The listing builds one solid part. Answer for the finished solid, in the listing's coordinates (mm). A direction names the side the tool comes from. Round coordinates to 2 decimals unless told otherwise and drop trailing zeros. Write each loop counter-clockwise with the first axis right and the second up, starting at its lowest first coordinate (ties: lowest second). Pieces come first, ordered by that corner, then holes. Notation, with made-up numbers: (45, 41) - (72, 41) arc R11 cw to (72, 50) - close; hole circle Ø11 at (-17.75, 24.5). An arc over 180 degrees is marked (long way). Return JSON: item names as keys, results as strings. Group by question number.
(1) Section B-B, the plane z = -3.25 is taken. Write down the section's boundary in (x, y), then the cut area to 3 significant figures.
(2) Determine the mould class of faces 3 (the flat face through (-12.45, -12.3, -0.14)), 4 (the flat face through (1, -54.428, -2)), 5 (the flat face through (41.704, 31, 0)), 6 (the cylindrical face through (-46.7, -3.73, 2.84)) for opening direction Y: +Y half, -Y half, draft (parallel to the pull), parting line (faces both ways), or undercut.
(3) Each of these flat-tipped pins is pushed along its axis until it touches: pin 1 (4 mm diameter, centred on x = 34.5, z = 0.5, fed in from -Y); pin 2 (1 mm diameter, centred on y = -4, z = 1.5, fed in from -X). Where does it stop, or does it pass through?
(4) Which of the six approach directions +Z, -Z, +X, -X, +Y, -Y give full straight-line access (tool end or side, diameter ignored) to faces 1 (the flat face through (-12.3, 12.45, -0.14)), 2 (the cylindrical face through (0.9, -52.73, 2.84))?
(5) Find the intervals of material crossed by line 1 along X through (y, z) = (32.5, -0.25); line 2 along Y through (x, z) = (3, 0); line 3 along Y through (x, z) = (34, 2.5), in increasing order. Write a range as [from, to].
(6) Section C-C, the plane x = 14 is taken. Write down the section's boundary in (y, z), then the cut area to 3 significant figures.
(7) Section A-A, the plane y = 0.5 is taken. Write down the section's boundary in (x, z).
```python
from build123d import *

# Parameters (mm, degrees)
F0_W        = 100
F0_H        = 100
F1_DEPTH    = 4
F3_T1_DEPTH = 124.4948974279
F3_T3_DEPTH = 124.4948974279
F5_DEPTH    = 25
F4_W        = 10
F4_H        = 10
F6_DEPTH    = 25
F7_DEPTH    = 4.4


# Not quite as in the source:
# - a fillet or chamfer that OpenCascade refuses, or shapes differently, is made with other operations: its cross-section is extruded or revolved along the edge and cut away or added


with BuildPart() as f1:
    # F0 (on Top) → F1 (new body)
    with BuildSketch(Plane.XY):
        with Locations((1.60311535, -4.4280775759)):
            Rectangle(F0_W, F0_H)
    extrude(amount=F1_DEPTH)

    # F3: fillet of radius 5 on 4 edges, made by hand

    # F3_s2 → F3_t1 (cut)
    with BuildSketch(Plane.YZ.offset(-60.6443333639)):
        with BuildLine():
            ThreePointArc((-54.4280775759, 0), (-52.6913757505, 2.8729833462), (-49.5290980903, 4))
            Line((-49.5290980903, 4), (-54.4280775759, 4))
            Line((-54.4280775759, 4), (-54.4280775759, 0))
        make_face()
        with BuildLine():
            ThreePointArc((45.5719224241, 0), (43.8352205987, 2.8729833462), (40.6729429385, 4))
            Line((40.6729429385, 4), (45.5719224241, 4))
            Line((45.5719224241, 4), (45.5719224241, 0))
        make_face()
    extrude(amount=F3_T1_DEPTH, mode=Mode.SUBTRACT)

    # F3_s4 → F3_t3 (cut)
    with BuildSketch(Plane.XZ.offset(-57.819371138)):
        with BuildLine():
            ThreePointArc((51.60311535, 0), (49.8664135246, 2.8729833462), (46.7041358644, 4))
            Line((46.7041358644, 4), (51.60311535, 4))
            Line((51.60311535, 4), (51.60311535, 0))
        make_face()
        with BuildLine():
            ThreePointArc((-48.39688465, 0), (-46.6601828246, 2.8729833462), (-43.4979051644, 4))
            Line((-43.4979051644, 4), (-48.39688465, 4))
            Line((-48.39688465, 4), (-48.39688465, 0))
        make_face()
    extrude(amount=F3_T3_DEPTH, mode=Mode.SUBTRACT)

    # F2 (on face) → F5 (cut)
    with BuildSketch(Plane.XY.offset(4)):
        Polygon((-7.2487373415, -17.5), (7.2487373415, -17.5), (17.5, -7.2487373415), (17.5, 7.2487373415), (7.2487373415, 17.5), (-7.2487373415, 17.5), (-17.5, 7.2487373415), (-17.5, -7.2487373415), align=None)
    extrude(amount=-F5_DEPTH, mode=Mode.SUBTRACT)

    # F4 (on face) → F6 (cut)
    with BuildSketch(Plane.XY.offset(4)):
        with Locations((36.7041358644, 30.6729429385)):
            Rectangle(F4_W, F4_H)
    extrude(amount=-F6_DEPTH, mode=Mode.SUBTRACT)

    # F7 (add): a face of the model
    f7_faces = [f1.faces().sort_by_distance(p)[0] for p in [
        (1.60311535, -53.0138640135, 0),
    ]]
    extrude(f7_faces, amount=F7_DEPTH)


solid = f1.part
```
Working result:
{
 "1": {"outline": "(-48.4, -54.43) - (51.6, -54.43) - (51.6, 45.57) - (-48.4, 45.57) - close; hole (-17.5, -7.25) - (-7.25, -17.5) - (7.25, -17.5) - (17.5, -7.25) - (17.5, 7.25) - (7.25, 17.5) - (-7.25, 17.5) - (-17.5, 7.25) - close; hole (31.7, 25.67) - (41.7, 25.67) - (41.7, 35.67) - (31.7, 35.67) - close", "area": "8,890 mm^2"},
 "2": {"face 3": "undercut", "face 4": "-Y half", "face 5": "undercut", "face 6": "draft"},
 "3": {"pin 1": "stops at y = -54.43", "pin 2": "stops at x = -48.08"},
 "4": {"face 1": "+Z, -Z", "face 2": "+Z, +X, -X, -Y"},
 "5": {"line 1": "x = [-48.4, 31.7], [41.7, 51.6]", "line 2": "y = [-54.43, -17.5], [17.5, 45.57]", "line 3": "y = [-53.1, 25.67], [35.67, 44.24]"},
 "6": {"outline": "(-54.43, -4.4) - (-10.75, -4.4) - (-10.75, 4) - (-49.53, 4) arc R5 ccw to (-54.43, 0) - close; (10.75, -4.4) - (45.57, -4.4) - (45.57, 0) arc R5 ccw to (40.67, 4) - (10.75, 4) - close", "area": "650 mm^2"},
 "7": {"outline": "(-48.4, -4.4) - (-17.5, -4.4) - (-17.5, 4) - (-43.5, 4) arc R5 ccw to (-48.4, 0) - close; (17.5, -4.4) - (51.6, -4.4) - (51.6, 0) arc R5 ccw to (46.7, 4) - (17.5, 4) - close"}
}
